Could you check a few things on this model? Use its own coordinates, in mm. Face numbers are marked on the shaded views. Give positions to 0.01 mm unless a question says otherwise; leave off trailing zeros. Loops run counter-clockwise (first coordinate to the right, second up) from the corner with the lowest first, then second, coordinate; pieces in that order, holes last. Notation, with made-up numbers: M -10,67 L -1,67 A23 ccw -1,103 Z; hole C -3.5,36.25 d1. An arc over 180 degrees is marked long. Answer in a Markdown table with one row per item. Add a question column.
1. If we section it at C-C on x = -15.5: Count the separate pieces of the cut face and the enclosed holes in it, then the cut area to 3 significant figures.
2. If we section it at B-B on x = -40.5: List the corners of the cut face in (y, z) for me.
3. If we section it at D-D on z = 30: List the corners of the cut face in (x, y) for me.
4. Thinking about a two-plate mould opening in Z: for the marked faces 1, 2, 3 and 4, which applies, released by +Z, released by -Z, zero draft, split by the parting line, or undercut?
5. I need wall thicknesses on line 1 along X through (y, z) = (39, -65.5); line 2 along Z through (x, y) = (-39.5, 64); line 3 along Z through (x, y) = (-15, 49.5). Which ranges of each line are inside material? Lowest first, please. Write a range as from..to.
6. If we section it at A-A on y = 33.5: List the corners of the cut face in (x, z) for me, then the cut area to 3 significant figures.
7. I'm going to push flat-ended pins straight in: pin 1 Ø6 at (x, y) = (-59, 15) entering from -Z; pin 2 Ø8 at (y, z) = (57.5, -18.5) entering from -X; pin 3 Ø10 at (y, z) = (23, 19) entering from -X. Where does each tip first touch, or does it pass through?
```python
from build123d import *

# Parameters (mm, degrees)
BOSS_EXTRUDE1_DEPTH = 86
CUT_EXTRUDE1_REACH  = 88
CUT_EXTRUDE2_START  = -4
CUT_EXTRUDE2_DEPTH  = 17.2
CUT_EXTRUDE3_START  = -65
CUT_EXTRUDE3_DEPTH  = 17
SKETCH5_W           = 12
SKETCH5_H           = 71
BOSS_EXTRUDE2_DEPTH = 45
SKETCH6_W           = 6
SKETCH6_H           = 71
CUT_EXTRUDE4_DEPTH  = 45
CUT_EXTRUDE6_REACH  = 89
SKETCH8_R           = 2.25
SKETCH9_R           = 3.25
CUT_EXTRUDE7_DEPTH  = 59.8792938
CUT_EXTRUDE8_START  = -6
CUT_EXTRUDE8_DEPTH  = 2.5
FILLET1_R           = 10
SKETCH11_W          = 7.611163598
SKETCH11_H          = 6
BOSS_EXTRUDE3_DEPTH = 45


with BuildPart() as part:
    # Sketch1 → Boss-Extrude1 (new body)
    with BuildSketch(Plane(origin=(0, 0, 0), x_dir=(1, 0, 0), z_dir=(0, 1, 0))):
        Polygon((-7.52701042, -41.304091879), (-7.52701042, 88.695908121), (-27.52701042, 88.695908121), (-27.52701042, 68.695908121), (-21.40630422, 68.695908121), (-21.40630422, -21.304091879), (-27.52701042, -21.304091879), (-27.52701042, -41.304091879), align=None)
    extrude(amount=BOSS_EXTRUDE1_DEPTH)

    # Sketch2 → Cut-Extrude1 (cut, up to next)
    with BuildSketch(Plane(origin=(0, 86, 0), x_dir=(1, 0, 0), z_dir=(0, 1, 0)), mode=Mode.PRIVATE) as cut_extrude1_sk1:
        with BuildLine():
            Line((-17.52701042, 83.945908121), (-27.52701042, 83.945908121))
            Line((-27.52701042, 83.945908121), (-27.52701042, 73.445908121))
            Line((-27.52701042, 73.445908121), (-17.52701042, 73.445908121))
            ThreePointArc((-17.52701042, 73.445908121), (-12.27701042, 78.695908121), (-17.52701042, 83.945908121))
        make_face()
    cut_extrude1_tool1 = extrude(cut_extrude1_sk1.sketch, amount=-CUT_EXTRUDE1_REACH, mode=Mode.PRIVATE) & part.part
    add(cut_extrude1_tool1.solids().sort_by_distance((-20.41673, 86, -78.695908))[0], mode=Mode.SUBTRACT)
    # Sketch2 → Cut-Extrude1 (cut, up to next)
    with BuildSketch(Plane(origin=(0, 86, 0), x_dir=(1, 0, 0), z_dir=(0, 1, 0)), mode=Mode.PRIVATE) as cut_extrude1_sk2:
        with BuildLine():
            Line((-17.52701042, -26.054091879), (-27.52701042, -26.054091879))
            Line((-27.52701042, -26.054091879), (-27.52701042, -36.554091879))
            Line((-27.52701042, -36.554091879), (-17.52701042, -36.554091879))
            ThreePointArc((-17.52701042, -36.554091879), (-12.27701042, -31.304091879), (-17.52701042, -26.054091879))
        make_face()
    cut_extrude1_tool2 = extrude(cut_extrude1_sk2.sketch, amount=-CUT_EXTRUDE1_REACH, mode=Mode.PRIVATE) & part.part
    add(cut_extrude1_tool2.solids().sort_by_distance((-20.41673, 86, 31.304092))[0], mode=Mode.SUBTRACT)

    # Sketch4 → Cut-Extrude2 (cut)
    with BuildSketch(Plane.XZ.offset(CUT_EXTRUDE2_START)):
        with BuildLine():
            Line((-27.52701042, 24.384091879), (-27.52701042, 38.224091879))
            Line((-27.52701042, 38.224091879), (-25.949301656, 37.435237497))
            ThreePointArc((-25.949301656, 37.435237497), (-25.514380306, 37.2775939), (-25.054874465, 37.224091879))
            Line((-25.054874465, 37.224091879), (-23.550164803, 37.224091879))
            ThreePointArc((-23.550164803, 37.224091879), (-22.812872449, 37.364952297), (-22.179435405, 37.767691894))
            Line((-22.179435405, 37.767691894), (-21.05701042, 38.824091879))
            Line((-21.05701042, 38.824091879), (-17.52701042, 38.824091879))
            ThreePointArc((-17.52701042, 38.824091879), (-10.00701042, 31.304091879), (-17.52701042, 23.784091879))
            Line((-17.52701042, 23.784091879), (-21.05701042, 23.784091879))
            Line((-21.05701042, 23.784091879), (-22.179435405, 24.840491864))
            ThreePointArc((-22.179435405, 24.840491864), (-22.812872449, 25.243231461), (-23.550164803, 25.384091879))
            Line((-23.550164803, 25.384091879), (-25.054874465, 25.384091879))
            ThreePointArc((-25.054874465, 25.384091879), (-25.514380306, 25.330589858), (-25.949301656, 25.172946261))
            Line((-25.949301656, 25.172946261), (-27.52701042, 24.384091879))
        make_face()
        with BuildLine():
            Line((-21.05701042, -86.240594633), (-17.52701042, -86.240594633))
            ThreePointArc((-17.52701042, -86.240594633), (-9.994667164, -78.708251377), (-17.52701042, -71.175908121))
            Line((-17.52701042, -71.175908121), (-21.05701042, -71.175908121))
            Line((-21.05701042, -71.175908121), (-22.179435405, -72.232308106))
            ThreePointArc((-22.179435405, -72.232308106), (-22.812872449, -72.635047703), (-23.550164803, -72.775908121))
            Line((-23.550164803, -72.775908121), (-25.054874465, -72.775908121))
            ThreePointArc((-25.054874465, -72.775908121), (-25.514380306, -72.7224061), (-25.949301656, -72.564762503))
            Line((-25.949301656, -72.564762503), (-27.52701042, -71.775908121))
            Line((-27.52701042, -71.775908121), (-27.52701042, -85.615908121))
            Line((-27.52701042, -85.615908121), (-25.926859801, -84.840694199))
            ThreePointArc((-25.926859801, -84.840694199), (-25.502199364, -84.691261302), (-25.054874465, -84.640594633))
            Line((-25.054874465, -84.640594633), (-23.550164803, -84.640594633))
            ThreePointArc((-23.550164803, -84.640594633), (-22.812872449, -84.781455051), (-22.179435405, -85.184194648))
            Line((-22.179435405, -85.184194648), (-21.05701042, -86.240594633))
        make_face()
    extrude(amount=-CUT_EXTRUDE2_DEPTH, mode=Mode.SUBTRACT)

    # Sketch4<2> → Cut-Extrude3 (cut)
    with BuildSketch(Plane.XZ.offset(CUT_EXTRUDE3_START)):
        with BuildLine():
            Line((-27.52701042, 24.384091879), (-27.52701042, 38.224091879))
            Line((-27.52701042, 38.224091879), (-25.949301656, 37.435237497))
            ThreePointArc((-25.949301656, 37.435237497), (-25.514380306, 37.2775939), (-25.054874465, 37.224091879))
            Line((-25.054874465, 37.224091879), (-23.550164803, 37.224091879))
            ThreePointArc((-23.550164803, 37.224091879), (-22.812872449, 37.364952297), (-22.179435405, 37.767691894))
            Line((-22.179435405, 37.767691894), (-21.05701042, 38.824091879))
            Line((-21.05701042, 38.824091879), (-17.52701042, 38.824091879))
            ThreePointArc((-17.52701042, 38.824091879), (-10.00701042, 31.304091879), (-17.52701042, 23.784091879))
            Line((-17.52701042, 23.784091879), (-21.05701042, 23.784091879))
            Line((-21.05701042, 23.784091879), (-22.179435405, 24.840491864))
            ThreePointArc((-22.179435405, 24.840491864), (-22.812872449, 25.243231461), (-23.550164803, 25.384091879))
            Line((-23.550164803, 25.384091879), (-25.054874465, 25.384091879))
            ThreePointArc((-25.054874465, 25.384091879), (-25.514380306, 25.330589858), (-25.949301656, 25.172946261))
            Line((-25.949301656, 25.172946261), (-27.52701042, 24.384091879))
        make_face()
        with BuildLine():
            Line((-21.05701042, -86.240594633), (-17.52701042, -86.240594633))
            ThreePointArc((-17.52701042, -86.240594633), (-9.994667164, -78.708251377), (-17.52701042, -71.175908121))
            Line((-17.52701042, -71.175908121), (-21.05701042, -71.175908121))
            Line((-21.05701042, -71.175908121), (-22.179435405, -72.232308106))
            ThreePointArc((-22.179435405, -72.232308106), (-22.812872449, -72.635047703), (-23.550164803, -72.775908121))
            Line((-23.550164803, -72.775908121), (-25.054874465, -72.775908121))
            ThreePointArc((-25.054874465, -72.775908121), (-25.514380306, -72.7224061), (-25.949301656, -72.564762503))
            Line((-25.949301656, -72.564762503), (-27.52701042, -71.775908121))
            Line((-27.52701042, -71.775908121), (-27.52701042, -85.615908121))
            Line((-27.52701042, -85.615908121), (-25.926859801, -84.840694199))
            ThreePointArc((-25.926859801, -84.840694199), (-25.502199364, -84.691261302), (-25.054874465, -84.640594633))
            Line((-25.054874465, -84.640594633), (-23.550164803, -84.640594633))
            ThreePointArc((-23.550164803, -84.640594633), (-22.812872449, -84.781455051), (-22.179435405, -85.184194648))
            Line((-22.179435405, -85.184194648), (-21.05701042, -86.240594633))
        make_face()
    extrude(amount=-CUT_EXTRUDE3_DEPTH, mode=Mode.SUBTRACT)

    # Sketch5 → Boss-Extrude2 (add)
    with BuildSketch(Plane(origin=(-21.40630422, 0, 0), x_dir=(0, 0, -1), z_dir=(1, 0, 0))):
        with Locations((1.695908121, 50.5)):
            Rectangle(SKETCH5_W, SKETCH5_H)
    extrude(amount=-BOSS_EXTRUDE2_DEPTH)

    # Sketch6 → Cut-Extrude4 (cut)
    with BuildSketch(Plane.ZY.offset(66.40630422)):
        with Locations((1.304091879, 50.5)):
            Rectangle(SKETCH6_W, SKETCH6_H)
    extrude(amount=-CUT_EXTRUDE4_DEPTH, mode=Mode.SUBTRACT)

    # Sketch8 → Cut-Extrude6 (cut, up to next)
    with BuildSketch(Plane.XY.offset(-1.695908121), mode=Mode.PRIVATE) as cut_extrude6_sk1:
        with Locations((-57.90630422, 25)):
            Circle(SKETCH8_R)
    cut_extrude6_tool1 = extrude(cut_extrude6_sk1.sketch, amount=-CUT_EXTRUDE6_REACH, mode=Mode.PRIVATE) & part.part
    add(cut_extrude6_tool1.solids().sort_by_distance((-57.906304, 25, -1.695908))[0], mode=Mode.SUBTRACT)
    # Sketch8 → Cut-Extrude6 (cut, up to next)
    with BuildSketch(Plane.XY.offset(-1.695908121), mode=Mode.PRIVATE) as cut_extrude6_sk2:
        with Locations((-57.90630422, 76)):
            Circle(SKETCH8_R)
    cut_extrude6_tool2 = extrude(cut_extrude6_sk2.sketch, amount=-CUT_EXTRUDE6_REACH, mode=Mode.PRIVATE) & part.part
    add(cut_extrude6_tool2.solids().sort_by_distance((-57.906304, 76, -1.695908))[0], mode=Mode.SUBTRACT)
    # Sketch8 → Cut-Extrude6 (cut, up to next)
    with BuildSketch(Plane.XY.offset(-1.695908121), mode=Mode.PRIVATE) as cut_extrude6_sk3:
        with Locations((-27.90630422, 25)):
            Circle(SKETCH8_R)
    cut_extrude6_tool3 = extrude(cut_extrude6_sk3.sketch, amount=-CUT_EXTRUDE6_REACH, mode=Mode.PRIVATE) & part.part
    add(cut_extrude6_tool3.solids().sort_by_distance((-27.906304, 25, -1.695908))[0], mode=Mode.SUBTRACT)
    # Sketch8 → Cut-Extrude6 (cut, up to next)
    with BuildSketch(Plane.XY.offset(-1.695908121), mode=Mode.PRIVATE) as cut_extrude6_sk4:
        with Locations((-27.90630422, 76)):
            Circle(SKETCH8_R)
    cut_extrude6_tool4 = extrude(cut_extrude6_sk4.sketch, amount=-CUT_EXTRUDE6_REACH, mode=Mode.PRIVATE) & part.part
    add(cut_extrude6_tool4.solids().sort_by_distance((-27.906304, 76, -1.695908))[0], mode=Mode.SUBTRACT)

    # Sketch9 → Cut-Extrude7 (cut, through all)
    with BuildSketch(Plane(origin=(-7.52701042, 0, 0), x_dir=(0, 0, -1), z_dir=(1, 0, 0))):
        with Locations((61.695908121, 33.5)):
            Circle(SKETCH9_R)
        with Locations((-14.304091879, 33.5)):
            Circle(SKETCH9_R)
        with Locations((-14.304091879, 73.5)):
            Circle(SKETCH9_R)
        with Locations((61.695908121, 73.5)):
            Circle(SKETCH9_R)
    extrude(amount=-CUT_EXTRUDE7_DEPTH, mode=Mode.SUBTRACT)

    # Sketch10 → Cut-Extrude8 (cut)
    with BuildSketch(Plane(origin=(0, 0, -7.695908121), x_dir=(-1, 0, 0), z_dir=(0, 0, -1)).offset(CUT_EXTRUDE8_START)):
        Polygon((61.40630422, 27.020725942), (57.90630422, 29.041451884), (54.40630422, 27.020725942), (54.40630422, 22.979274058), (57.90630422, 20.958548116), (61.40630422, 22.979274058), align=None)
        Polygon((61.40630422, 78.020725942), (57.90630422, 80.041451884), (54.40630422, 78.020725942), (54.40630422, 73.979274058), (57.90630422, 71.958548116), (61.40630422, 73.979274058), align=None)
        Polygon((24.40630422, 22.979274058), (27.90630422, 20.958548116), (31.40630422, 22.979274058), (31.40630422, 27.020725942), (27.90630422, 29.041451884), (24.40630422, 27.020725942), align=None)
        Polygon((27.795986428, 71.960054045), (31.349841151, 73.884489013), (31.460158942, 77.924434968), (28.016622011, 80.039945955), (24.462767289, 78.115510987), (24.352449497, 74.075565032), align=None)
    extrude(amount=CUT_EXTRUDE8_DEPTH, mode=Mode.SUBTRACT)

    # Fillet1
    fillet1_edges = [part.edges().sort_by_distance(p)[0] for p in [
        (-66.40630422, 86, -4.695908121),
        (-66.40630422, 15, -4.695908121),
    ]]
    fillet(fillet1_edges, radius=FILLET1_R)

    # Sketch11 → Boss-Extrude3 (add)
    with BuildSketch(Plane.ZY.offset(21.40630422)):
        with Locations((2.109673678, 50.5)):
            Rectangle(SKETCH11_W, SKETCH11_H)
    extrude(amount=BOSS_EXTRUDE3_DEPTH)


solid = part.part
```
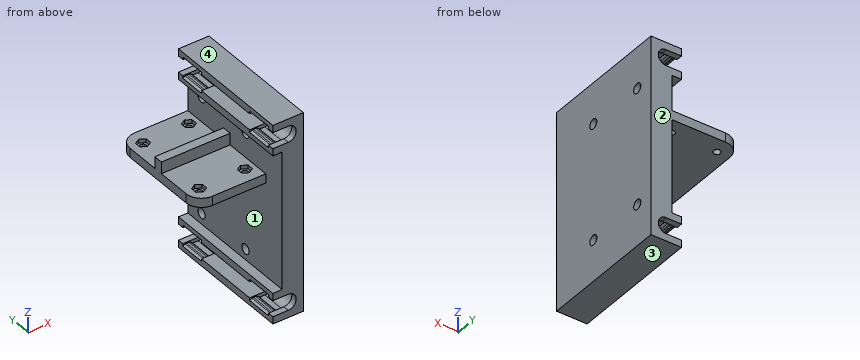
Results:
| question | item | result |
|---|---|---|
| 1 | separate pieces | 3 |
| 1 | enclosed holes | 4 |
| 1 | area | 9,050 mm2 |
| 2 | outline | M 15,-7.7 L 86,-7.7 L 86,-1.7 L 53.5,-1.7 L 53.5,5.92 L 47.5,5.92 L 47.5,-1.7 L 15,-1.7 Z |
| 3 | outline | M -12.44,0 L -7.53,0 L -7.53,86 L -12.44,86 L -12.44,82 L -10.12,82 L -10.12,65 L -12.44,65 L -12.44,21.2 L -10.12,21.2 L -10.12,4 L -12.44,4 Z |
| 4 | face 1 | undercut |
| 4 | face 2 | zero draft |
| 4 | face 3 | released by -Z |
| 4 | face 4 | released by +Z |
| 5 | line 1 | -21.41..-7.53 |
| 5 | line 2 | -7.7..-1.7 |
| 5 | line 3 | -88.7..-83.3, -74.09..26.7, 35.91..41.3 |
| 6 | outline | M -66.41,-7.7 L -21.41,-7.7 L -21.41,-58.45 L -7.53,-58.45 L -7.53,11.05 L -21.41,11.05 L -21.41,-1.7 L -66.41,-1.7 Z; M -27.53,-88.7 L -7.53,-88.7 L -7.53,-64.95 L -21.41,-64.95 L -21.41,-68.7 L -27.53,-68.7 L -27.53,-73.45 L -17.53,-73.45 A5.25 cw -17.53,-83.95 L -27.53,-83.95 Z; M -27.53,21.3 L -21.41,21.3 L -21.41,17.55 L -7.53,17.55 L -7.53,41.3 L -27.53,41.3 L -27.53,36.55 L -17.53,36.55 A5.25 cw -17.53,26.05 L -27.53,26.05 Z |
| 6 | area | 1,840 mm2 |
| 7 | pin 1 | z = -7.7 |
| 7 | pin 2 | x = -21.41 |
| 7 | pin 3 | x = -27.53 |
